```python
from build123d import *

# Parameters (mm, degrees)
SKETCH1_W           = 9.906
SKETCH1_H           = 30.48
BOSS_EXTRUDE1_DEPTH = 2.54
SKETCH2_W           = 5.08
SKETCH2_H           = 5.08
BOSS_EXTRUDE2_DEPTH = 3.429
SKETCH3_R           = 1.778
CUT_EXTRUDE1_DEPTH  = 12.7


with BuildPart() as part:
    # Sketch1 → Boss-Extrude1 (new body)
    with BuildSketch(Plane.XY):
        with Locations((-4.953, -15.24)):
            Rectangle(SKETCH1_W, SKETCH1_H)
    extrude(amount=BOSS_EXTRUDE1_DEPTH)

    # Sketch2 → Boss-Extrude2 (add)
    with BuildSketch(Plane.XY.offset(2.54)):
        with Locations((-4.953, -2.54)):
            Rectangle(SKETCH2_W, SKETCH2_H)
        with Locations((-4.953, -27.94)):
            Rectangle(SKETCH2_W, SKETCH2_H)
    extrude(amount=BOSS_EXTRUDE2_DEPTH)

    # Sketch3 → Cut-Extrude1 (cut)
    with BuildSketch(Plane.XY.offset(5.969)):
        with Locations((-4.953, -27.94)):
            Circle(SKETCH3_R)
        with Locations((-4.953, -2.54)):
            Circle(SKETCH3_R)
    extrude(amount=-CUT_EXTRUDE1_DEPTH, mode=Mode.SUBTRACT)


solid = part.part
```
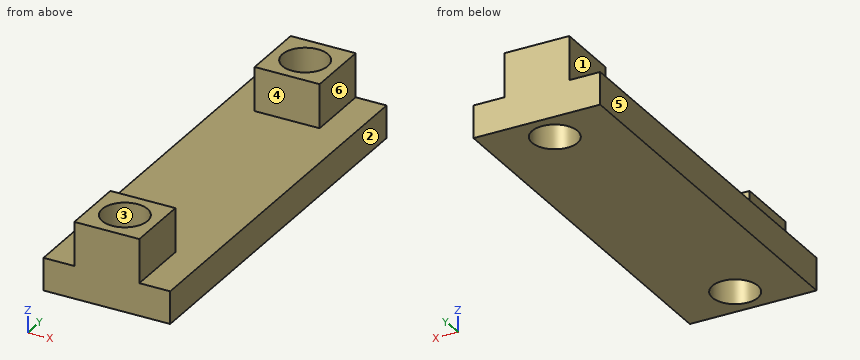
Work out the finished part from the listing and answer in its coordinate system (mm). Face numbers are marked on the shaded views. A direction names the side the tool comes from. Give positions to 0.01 mm unless a question says otherwise; leave off trailing zeros. Order: outer loops, then holes, each group sorted by start corner. A loop starts at its lowest first (then second) coordinate and runs counter-clockwise, first axis right, second up. Notation, with made-up numbers: (-17.5, 0) - (9.5, 0) arc R26 cw to (9.5, 32) - close; hole circle Ø8 at (81, 86.25). An arc over 180 degrees is marked (long way). One line per item, written item: value. Start each with the question number.
1. Section D-D, the plane z = 2.2 is taken. Write down the section's boundary in (x, y) (3 decimals), then the cut area to 3 significant figures.
2. Section A-A, the plane z = 4.3 is taken. Write down the section's boundary in (x, y) (3 decimals).
3. Section B-B, the plane y = -2.54 is taken. Write down the section's boundary in (x, z) (3 decimals).
4. For a pull along X with two mould halves and no side action, classify the marked faces 1, 2 and 3 as released by +X, released by -X, zero draft, split by the parting line, or undercut.
5. Which of the six approach directions +Z, -Z, +X, -X, +Y, -Y give full straight-line access (tool end or side, diameter ignored) to the marked faces 4, 5 and 6?
6. Each of these flat-tipped pins is pushed along its axis until it touches: pin 1 Ø1.5 at (x, z) = (-8.5, 4) entering from -Y; pin 2 Ø5 at (x, y) = (-5, -14.5) entering from +Z; pin 3 Ø1.7 at (y, z) = (-3, 4) entering from +X; pin 4 Ø1.7 at (y, z) = (-2.5, 4) entering from -X. Where does it stop, or does it pass through?
7. Consider line 1 (Y direction, x = -3, z = 4.1); line 2 (Z direction, x = -0.75, y = -3); line 3 (X direction, y = -2.5, z = 4.35). Determine where each line is inside the solid, lowest interval first.
8. Section C-C, the plane x = -6.25 is taken. Write down the section's boundary in (y, z), then the cut area to 3 significant figures.
Filled sheet:
1. outline: (-9.906, -30.48) - (0, -30.48) - (0, 0) - (-9.906, 0) - close; hole circle Ø3.556 at (-4.953, -27.94); hole circle Ø3.556 at (-4.953, -2.54)
1. area: 282 mm²
2. outline: (-7.493, -30.48) - (-2.413, -30.48) - (-2.413, -25.4) - (-7.493, -25.4) - close; (-7.493, -5.08) - (-2.413, -5.08) - (-2.413, 0) - (-7.493, 0) - close; hole circle Ø3.556 at (-4.953, -27.94); hole circle Ø3.556 at (-4.953, -2.54)
3. outline: (-9.906, 0) - (-6.731, 0) - (-6.731, 5.969) - (-7.493, 5.969) - (-7.493, 2.54) - (-9.906, 2.54) - close; (-3.175, 0) - (0, 0) - (0, 2.54) - (-2.413, 2.54) - (-2.413, 5.969) - (-3.175, 5.969) - close
4. face 1: released by -X
4. face 2: released by +X
4. face 3: undercut
5. face 4: +Z, +X, -X
5. face 5: +Z, -Z, -X, +Y, -Y
5. face 6: +Z, +X, +Y, -Y
6. pin 1: through
6. pin 2: z = 2.54
6. pin 3: x = -2.41
6. pin 4: x = -7.49
7. line 1: -30.48 to -25.4, -5.08 to 0
7. line 2: 0 to 2.54
7. line 3: -7.49 to -6.73, -3.18 to -2.41
8. outline: (-30.48, 0) - (-29.16, 0) - (-29.16, 5.97) - (-30.48, 5.97) - close; (-26.72, 0) - (-3.76, 0) - (-3.76, 5.97) - (-5.08, 5.97) - (-5.08, 2.54) - (-25.4, 2.54) - (-25.4, 5.97) - (-26.72, 5.97) - close; (-1.32, 0) - (0, 0) - (0, 5.97) - (-1.32, 5.97) - close
8. area: 83.2 mm²
